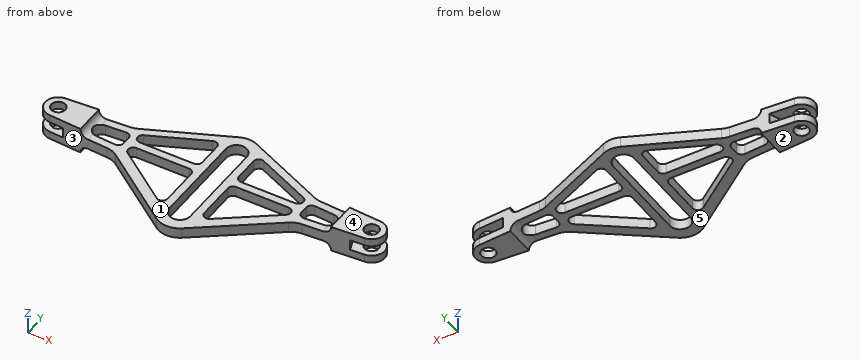
```python
from build123d import *

# Parameters (mm, degrees)
BOSS_EXTRUDE1_DEPTH                    = 12.5
SKETCH2_W                              = 240
SKETCH2_H                              = 181.658858688
CUT_EXTRUDE1_DEPTH                     = 7.5
F_13_5_13_5_DIAMETER_HOLE1_D           = 13.5
F_13_5_13_5_DIAMETER_HOLE1_CSINK_D     = 13.55
F_13_5_13_5_DIAMETER_HOLE1_CSINK_ANGLE = 90
CUT_EXTRUDE2_DEPTH                     = 5
FILLET1_R                              = 7.5
FILLET2_R                              = 20
CUT_EXTRUDE3_DEPTH                     = 181.166481325
CUT_EXTRUDE4_DEPTH                     = 181.166481325
CUT_EXTRUDE5_DEPTH                     = 181.166481325


with BuildPart() as part:
    # Sketch1 → Boss-Extrude1 (new, symmetric)
    with BuildSketch(Plane.XY):
        with BuildLine():
            Line((-150.817539115, 12.47323654), (-87.5, 16.623287311))
            Line((-87.5, 16.623287311), (-8.098559617, 51.78697165))
            ThreePointArc((-8.098559617, 51.78697165), (0, 53.5), (8.098559617, 51.78697165))
            Line((8.098559617, 51.78697165), (87.5, 16.623287311))
            Line((87.5, 16.623287311), (150.817539115, 12.47323654))
            ThreePointArc((150.817539115, 12.47323654), (162.5, 0), (150.817539115, -12.47323654))
            Line((150.817539115, -12.47323654), (87.5, -16.623287311))
            Line((87.5, -16.623287311), (12.310141778, -71.78094771))
            ThreePointArc((12.310141778, -71.78094771), (0, -75.812010875), (-12.310141778, -71.78094771))
            Line((-12.310141778, -71.78094771), (-87.5, -16.623287311))
            Line((-87.5, -16.623287311), (-150.817539115, -12.47323654))
            ThreePointArc((-150.817539115, -12.47323654), (-162.5, 0), (-150.817539115, 12.47323654))
        make_face()
    extrude(amount=BOSS_EXTRUDE1_DEPTH, both=True)

    # Sketch2 → Cut-Extrude1 (cut)
    with BuildSketch(Plane.XY.offset(12.5)):
        Rectangle(SKETCH2_W, SKETCH2_H)
    cut_extrude1 = extrude(amount=-CUT_EXTRUDE1_DEPTH, mode=Mode.SUBTRACT)

    # Mirror2: Cut-Extrude1 across plane
    add(cut_extrude1.mirror(Plane.XY), mode=Mode.SUBTRACT)

    # Ø13.5 (13.5) Diameter Hole1 (through all)
    with Locations(Plane.XY.offset(12.5)):
        with Locations((-150, 0), (150, 0)):
            CounterSinkHole(F_13_5_13_5_DIAMETER_HOLE1_D / 2, F_13_5_13_5_DIAMETER_HOLE1_CSINK_D / 2, counter_sink_angle=F_13_5_13_5_DIAMETER_HOLE1_CSINK_ANGLE)

    # Sketch5 → Cut-Extrude2 (cut, symmetric)
    with BuildSketch(Plane.XY):
        with BuildLine():
            Line((-137.5, -13.34611417), (-127.54739536, 13.998442342))
            Line((-127.54739536, 13.998442342), (-150.817539115, 12.47323654))
            ThreePointArc((-150.817539115, 12.47323654), (-162.5, 0), (-150.817539115, -12.47323654))
            Line((-150.817539115, -12.47323654), (-137.5, -13.34611417))
        make_face()
    cut_extrude2 = extrude(amount=CUT_EXTRUDE2_DEPTH, both=True, mode=Mode.SUBTRACT)

    # Mirror3: Cut-Extrude2 across plane
    add(cut_extrude2.mirror(Plane(origin=(0, 0, 0), x_dir=(0, 0, 1), z_dir=(1, 0, 0))), mode=Mode.SUBTRACT)

    # Fillet1
    fillet1_edges = [part.edges().sort_by_distance(p)[0] for p in [
        (120, 0, -5),
        (120, 0, 5),
        (-120, 0, -5),
        (-120, 0, 5),
    ]]
    fillet(fillet1_edges, radius=FILLET1_R - 0.0001)  # a hair under: the kernel refuses the full size

    # Fillet2
    fillet2_edges = [part.edges().sort_by_distance(p)[0] for p in [
        (-87.5, 16.623287311, 0),
        (87.5, 16.623287311, 0),
        (87.5, -16.623287311, 0),
        (-87.5, -16.623287311, 0),
    ]]
    fillet(fillet2_edges, radius=FILLET2_R)

    # Sketch6 → Cut-Extrude3 (cut, through all)
    with BuildSketch(Plane.XY.offset(5)):
        with BuildLine():
            Line((10, 33.5), (10, -55))
            ThreePointArc((10, -55), (0, -65), (-10, -55))
            Line((-10, -55), (-10, 33.5))
            ThreePointArc((-10, 33.5), (0, 43.5), (10, 33.5))
        make_face()
    extrude(amount=-CUT_EXTRUDE3_DEPTH, mode=Mode.SUBTRACT)

    # Sketch7 → Cut-Extrude4 (cut, through all)
    with BuildSketch(Plane.XY.offset(5)):
        with BuildLine():
            Line((76.433247958, 13.321742913), (24.524639904, 36.309964527))
            ThreePointArc((24.524639904, 36.309964527), (19.772656927, 35.928877859), (17.5, 31.738221615))
            Line((17.5, 31.738221615), (17.5, 8.75))
            ThreePointArc((17.5, 8.75), (18.964466094, 5.214466094), (22.5, 3.75))
            Line((22.5, 3.75), (74.408608053, 3.75))
            ThreePointArc((74.408608053, 3.75), (79.300372283, 7.715281334), (76.433247958, 13.321742913))
        make_face()
        with BuildLine():
            Line((75.830583045, -12.781553657), (25.457460923, -49.734191007))
            ThreePointArc((25.457460923, -49.734191007), (20.240277076, -50.162867423), (17.5, -45.70263735))
            Line((17.5, -45.70263735), (17.5, -8.75))
            ThreePointArc((17.5, -8.75), (18.964466094, -5.214466094), (22.5, -3.75))
            Line((22.5, -3.75), (72.873122122, -3.75))
            ThreePointArc((72.873122122, -3.75), (77.624846456, -7.194006473), (75.830583045, -12.781553657))
        make_face()
    cut_extrude4 = extrude(amount=-CUT_EXTRUDE4_DEPTH, mode=Mode.SUBTRACT)

    # Mirror4: Cut-Extrude4 across plane
    add(cut_extrude4.mirror(Plane(origin=(0, 0, 0), x_dir=(0, 0, 1), z_dir=(1, 0, 0))), mode=Mode.SUBTRACT)

    # Sketch8 → Cut-Extrude5 (cut, symmetric)
    with BuildSketch(Plane.XY.offset(5)):
        with BuildLine():
            Line((-109.308995171, 7.677757716), (-90.327015646, 8.921902385))
            ThreePointArc((-90.327015646, 8.921902385), (-86.58203849, 7.581928132), (-85, 3.932607769))
            Line((-85, 3.932607769), (-85, -3.932607769))
            ThreePointArc((-85, -3.932607769), (-86.58203849, -7.581928132), (-90.327015646, -8.921902385))
            Line((-90.327015646, -8.921902385), (-109.308995171, -7.677757716))
            ThreePointArc((-109.308995171, -7.677757716), (-116.5, 0), (-109.308995171, 7.677757716))
        make_face()
    cut_extrude5 = extrude(amount=CUT_EXTRUDE5_DEPTH, both=True, mode=Mode.SUBTRACT)

    # Mirror5: Cut-Extrude5 across plane
    add(cut_extrude5.mirror(Plane(origin=(0, 0, 0), x_dir=(0, 0, 1), z_dir=(1, 0, 0))), mode=Mode.SUBTRACT)


solid = part.part
```
Could you check a few things on this model? Use its own coordinates, in mm. Face numbers are marked on the shaded views. A direction names the side the tool comes from. Coordinates: 2 decimals unless noted, no trailing zeros. Write each loop counter-clockwise with the first axis right and the second up, starting at its lowest first coordinate (ties: lowest second). Pieces come first, ordered by that corner, then holes. Notation, with made-up numbers: (68, -30.5) -> (84, -30.5) arc R24 ccw to (84, 2.5) -> close; hole circle Ø9 at (71, -14). An arc over 180 degrees is marked (long way). One line per question, with ' | ' between items. Start each with the question number.
1. Thinking about a two-plate mould opening in X: for the marked faces 1, 2 and 3, which applies, pulls with the +X half, pulls with the -X half, needs draft (parallel to the pull), parting line crosses it, or undercut?
2. If we section it at C-C (y = 28.5): Please give me the cut outline in (x, z).
3. If we section it at B-B (z = -9): Please give me the cut outline in (x, y).
4. For the marked faces 4 and 5, which set-ups out of +Z, -Z, +X, -X, +Y, -Y let a thin tool reach every point of the face, with its end or its side?
5. Please list where these lines run through material, in increasing order: line 1 along Y through (x, z) = (-150, 8.5); line 2 along X through (y, z) = (0, 9.5); line 3 along X through (y, z) = (0, 9.75).
6. If we section it at A-A (x = 0): Please give me the cut outline in (y, z), and give its area (3 significant figures).
7. If we section it at D-D (y = 0): Count the separate pieces of the cut face and the enclosed holes in it, and give its area (3 significant figures).
8. Will these pins go through, and if not, where does the flat tip stop? P1, Ø11, axis at x = -150, y = 0, coming from the +Z side; P2, Ø5, axis at y = -32.5, z = 2.5, coming from the -X side; P3, Ø2.5, axis at y = 0, z = 0.5, coming from the -X side; P4, Ø8, axis at y = -31, z = -1, coming from the +X side.
Return value:
1) face 1: undercut | face 2: needs draft | face 3: pulls with the -X half
2) outline: (-60.68, -5) -> (-42.16, -5) -> (-42.16, 5) -> (-60.68, 5) -> close; (-17.5, -5) -> (-10, -5) -> (-10, 5) -> (-17.5, 5) -> close; (10, -5) -> (17.5, -5) -> (17.5, 5) -> (10, 5) -> close; (42.16, -5) -> (60.68, -5) -> (60.68, 5) -> (42.16, 5) -> close
3) outline: (-150.82, -12.47) -> (-119.13, -14.55) -> (-119.13, 14.55) -> (-150.82, 12.47) arc R12.5 ccw to start; (119.13, -14.55) -> (150.82, -12.47) arc R12.5 ccw to (150.82, 12.47) -> (119.13, 14.55) -> close; hole circle Ø13.5 at (-150, 0); hole circle Ø13.5 at (150, 0)
4) face 4: +Z, +X, -X, +Y, -Y | face 5: -Z, +Y, -Y
5) line 1: y = -12.53 to -6.75, 6.75 to 12.53 | line 2: x = -162.5 to -156.75, -143.25 to -119.37, 119.37 to 143.25, 156.75 to 162.5 | line 3: x = -162.5 to -156.75, -143.25 to -119.48, 119.48 to 143.25, 156.75 to 162.5
6) outline: (-75.81, -5) -> (-65, -5) -> (-65, 5) -> (-75.81, 5) -> close; (43.5, -5) -> (53.5, -5) -> (53.5, 5) -> (43.5, 5) -> close | area: 208 mm²
7) separate pieces: 8 | enclosed holes: 0 | area: 2,740 mm²
8) P1: passes through | P2: stops at x = -69.27 | P3: stops at x = -133.1 | P4: stops at x = 73.35
